Can you work these out from the model? Positions are in its coordinate system, mm. Face numbers are marked on the shaded views. Round coordinates to 2 decimals unless told otherwise and drop trailing zeros. Write each loop counter-clockwise with the first axis right and the second up, starting at its lowest first coordinate (ties: lowest second). Pieces come first, ordered by that corner, then holes. Notation, with made-up numbers: (70.5, 76.25) - (79.5, 76.25) arc R13 cw to (79.5, 88.25) - close; hole circle Ø4 at (64.25, -10.75). An arc over 180 degrees is marked (long way). One line per item, written item: value. Start each with the question number.
(1) I want a section at A-A on x = 76.5. List the corners of the cut face in (y, z) for me, plus the area to 3 significant figures.
(2) Thinking about a two-plate mould opening in X: for the marked faces 1, 2 and 3, which applies, +X half, -X half, draft (parallel to the pull), parting line (faces both ways), or undercut?
(3) I want a section at B-B on y = 24.5. List the corners of the cut face in (x, z) for me, plus the area to 4 significant figures.
(4) I'm going to push flat-ended pins straight in: pin 1 Ø1 at (x, z) = (20.5, 12.5) entering from -Y; pin 2 Ø6 at (x, z) = (-29.5, 12) entering from -Y; pin 3 Ø1.5 at (x, y) = (49, -25) entering from -Z; pin 4 Ø1 at (x, z) = (-42.5, 4.5) entering from -Y. Where does each tip first touch, or does it pass through?
(5) I want a section at D-D on y = 92. List the corners of the cut face in (x, z) for me, plus the area to 3 significant figures.
(6) If I drill on L1, parallel to Y at x = 37, z = 6.75; L2, parallel to Y at x = -19.5, z = 3.5; L3, parallel to X at y = -66, z = 11, over which ranges is the centre line in solid material (lowest first)? Write a range as from..to.
(7) I want a section at C-C on z = 15. List the corners of the cut face in (x, y) for me, plus the area to 3 significant figures.
from build123d import *

# Parameters (mm, degrees)
PRISM001_DEPTH = 19
PRISM_DEPTH    = 19


with BuildPart() as prism001:
    # Prism001 → Prism001 (new body)
    with BuildSketch(Plane.XY):
        Polygon((95, 0), (-47.5, 82.272413), (-47.5, -82.272413), align=None)
    extrude(amount=PRISM001_DEPTH)


with BuildPart() as cut:
    # Prism → Prism (new body)
    with BuildSketch(Plane.XY):
        Polygon((165, 0), (-82.5, 142.894192), (-82.5, -142.894192), align=None)
    extrude(amount=PRISM_DEPTH)

    # Cut: cut Prism001
    add(prism001.part, mode=Mode.SUBTRACT)


solid = cut.part
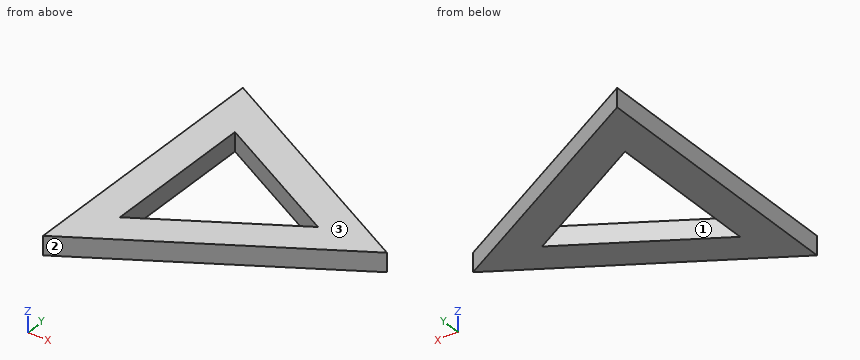
Established:
1. outline: (-51.1, 0) - (-10.68, 0) - (-10.68, 19) - (-51.1, 19) - close; (10.68, 0) - (51.1, 0) - (51.1, 19) - (10.68, 19) - close
1. area: 1,540 mm2
2. face 1: undercut
2. face 2: +X half
2. face 3: draft
3. outline: (-82.5, 0) - (-47.5, 0) - (-47.5, 19) - (-82.5, 19) - close; (52.56, 0) - (122.56, 0) - (122.56, 19) - (52.56, 19) - close
3. area: 1,995 mm2
4. pin 1: y = -83.72
4. pin 2: y = -114.03
4. pin 3: through
4. pin 4: y = -120.09
5. outline: (-82.5, 0) - (5.65, 0) - (5.65, 19) - (-82.5, 19) - close
5. area: 1,670 mm2
6. L1: -73.9..-33.49, 33.49..73.9
6. L2: -106.52..-66.11, 66.11..106.52
6. L3: -82.5..-47.5, -19.32..50.68
7. outline: (-82.5, -142.89) - (165, 0) - (-82.5, 142.89) - close; hole (-47.5, -82.27) - (95, 0) - (-47.5, 82.27) - close
7. area: 23,600 mm2
